Design review of the part built by this model. Coordinates are the model's own, in mm. A direction names the side the tool comes from. Give positions to 0.01 mm unless a question says otherwise; leave off trailing zeros. Write each loop counter-clockwise with the first axis right and the second up, starting at its lowest first coordinate (ties: lowest second). Pieces come first, ordered by that corner, then holes. Notation, with made-up numbers: M -22,39 L -2,39 A20 cw -2,65 Z; hole C 17.5,25 d7. An arc over 180 degrees is marked long. Use a Markdown table: item, result. Add a question column.
```python
from build123d import *

# Parameters (mm, degrees)
SKETCH1_W               = 21
SKETCH1_H               = 157
BOSS_EXTRUDE1_DEPTH     = 1.7
BOSS_EXTRUDE2_DEPTH     = 1.3
SKETCH3_R               = 1.75
CUT_EXTRUDE1_DEPTH      = 4
CUT_EXTRUDE2_DEPTH      = 1
CUT_EXTRUDE2_DEPTH_BACK = 4


with BuildPart() as part:
    # Sketch1 → Boss-Extrude1 (new body)
    with BuildSketch(Plane.XY):
        Rectangle(SKETCH1_W, SKETCH1_H)
    extrude(amount=BOSS_EXTRUDE1_DEPTH)

    # Sketch2 → Boss-Extrude2 (add)
    with BuildSketch(Plane(origin=(0, 0, 0), x_dir=(-1, 0, 0), z_dir=(0, 0, -1))):
        Polygon((-5.5, 78.5), (-5.5, -78.5), (10.5, -78.5), (10.5, 78.5), (-1.5, 78.5), (-1.5, 82.5), (-5.5, 82.5), align=None)
    extrude(amount=BOSS_EXTRUDE2_DEPTH)

    # Sketch3 → Cut-Extrude1 (cut, through all)
    with BuildSketch(Plane.XY.offset(1.7)):
        with Locations((-3, 54.5)):
            Circle(SKETCH3_R)
        with Locations((-3, -7)):
            Circle(SKETCH3_R)
        with Locations((-3, -68.5)):
            Circle(SKETCH3_R)
    extrude(amount=-CUT_EXTRUDE1_DEPTH, mode=Mode.SUBTRACT)

    # Sketch4 → Cut-Extrude2 (cut, two sides)
    with BuildSketch(Plane.XY.offset(1.7)) as cut_extrude2_sk:
        Polygon((5.499288315, -78.5), (10.5, -68.500735895), (10.5, -78.5), align=None)
    extrude(amount=CUT_EXTRUDE2_DEPTH, mode=Mode.SUBTRACT)
    extrude(cut_extrude2_sk.sketch, amount=-CUT_EXTRUDE2_DEPTH_BACK, mode=Mode.SUBTRACT)


solid = part.part
```
(1) Add section A-A on y = -7. Give the boundary of the cut face in (x, z), then the cut area to 3 significant figures.
(2) Machinability: for faces 1 (the flat face through (-2, 3, -1.3)), 2 (the flat face through (4, 81, 0)), which of the approach directions +Z, -Z, +X, -X, +Y, -Y give a long, thin tool a straight path to every point of the face, cutting with its end or side? Answer none if there is none.
(3) The part is to be moulded in two halves that separate along X. For faces 3 (the flat face through (7.965, -73.57, 0.888)), 4 (the cylindrical face through (-2.19, -8.55, 0.22)), 5 (the flat face through (8, 1, 0)), say which applies: released by +X, released by -X, zero draft, split by the parting line, or undercut.
(4) Wall thickness on L1, parallel to Y at x = -3, z = 0.65; L2, parallel to Y at x = -4.5, z = 1.15; L3, parallel to Y at x = -7, z = 0.55: over which ranges is each line inside the solid? List them lowest first.
(5) For pin 1 (0.9 mm diameter, centred on x = -1.5, z = 0.5, fed in from +Y); pin 2 (0.6 mm diameter, centred on y = 81, z = -1, fed in from -X); pin 3 (4 mm diameter, centred on x = -3, y = 54.5, fed in from +Z); pin 4 (2.5 mm diameter, centred on x = 9, y = -35, fed in from -Z), all flat-tipped, find the tip position at first contact; note any pin that passes through.
(6) Add section C-C on z = 0.95. Give the boundary of the cut face in (x, y).
(7) Add section B-B on x = -3. Give the boundary of the cut face in (y, z).
(8) Add section D-D on y = 68.5. Give the boundary of the cut face in (x, z).
From the geometry:
| question | item | result |
|---|---|---|
| 1 | outline | M -10.5,-1.3 L -4.75,-1.3 L -4.75,1.7 L -10.5,1.7 Z; M -1.25,-1.3 L 5.5,-1.3 L 5.5,0 L 10.5,0 L 10.5,1.7 L -1.25,1.7 Z |
| 1 | area | 46.0 mm^2 |
| 2 | face 1 | -Z, +X, -X, +Y, -Y |
| 2 | face 2 | +Z, +X, -X, +Y |
| 3 | face 3 | released by +X |
| 3 | face 4 | undercut |
| 3 | face 5 | zero draft |
| 4 | L1 | y = -78.5 to -70.25, -66.75 to -8.75, -5.25 to 52.75, 56.25 to 78.5 |
| 4 | L2 | y = -78.5 to -69.4, -67.6 to -7.9, -6.1 to 53.6, 55.4 to 78.5 |
| 4 | L3 | y = -78.5 to 78.5 |
| 5 | pin 1 | stops at y = 78.5 |
| 5 | pin 2 | stops at x = 1.5 |
| 5 | pin 3 | stops at z = 1.7 |
| 5 | pin 4 | stops at z = 0 |
| 6 | outline | M -10.5,-78.5 L 5.5,-78.5 L 10.5,-68.5 L 10.5,78.5 L -10.5,78.5 Z; hole C -3,-68.5 d3.5; hole C -3,-7 d3.5; hole C -3,54.5 d3.5 |
| 7 | outline | M -78.5,-1.3 L -70.25,-1.3 L -70.25,1.7 L -78.5,1.7 Z; M -66.75,-1.3 L -8.75,-1.3 L -8.75,1.7 L -66.75,1.7 Z; M -5.25,-1.3 L 52.75,-1.3 L 52.75,1.7 L -5.25,1.7 Z; M 56.25,-1.3 L 78.5,-1.3 L 78.5,1.7 L 56.25,1.7 Z |
| 8 | outline | M -10.5,-1.3 L 5.5,-1.3 L 5.5,0 L 10.5,0 L 10.5,1.7 L -10.5,1.7 Z |
